```python
from build123d import *

# Parameters (mm, degrees)
BOSS_EXTRUDE1_DEPTH     = 3.7
CHAMFER1_SIZE           = 0.9
CHAMFER1_SIZE2          = 2
CHAMFER2_SIZE           = 2
CHAMFER2_SIZE2          = 0.9
CHAMFER4_SIZE           = 0.9
CHAMFER4_SIZE2          = 2
CHAMFER5_SIZE           = 2
CHAMFER5_SIZE2          = 0.9
CUT_EXTRUDE2_DEPTH      = 1
CUT_EXTRUDE2_DEPTH_BACK = 4.7
CUT_EXTRUDE4_DEPTH      = 1
CUT_EXTRUDE4_DEPTH_BACK = 4.7


with BuildPart() as part:
    # Sketch1 → Boss-Extrude1 (new body)
    with BuildSketch(Plane.XY):
        Polygon((2.936521739, 23.386304348), (2.936521739, -12.613695652), (-3.203478261, -17.151956522), (-3.203478261, 18.848043478), align=None)
    extrude(amount=BOSS_EXTRUDE1_DEPTH)

    # Chamfer1
    chamfer1_edges = [part.edges().sort_by_distance(p)[0] for p in [
        (-0.133478261, 21.117173913, 3.7),
    ]]
    chamfer1_side = [part.faces().sort_by_distance(p)[0] for p in [
        (-0.133478261, 21.117173913, 1.85),
    ]]
    chamfer(chamfer1_edges, length=CHAMFER1_SIZE, length2=CHAMFER1_SIZE2, reference=chamfer1_side[0])

    # Chamfer2
    chamfer2_edges = [part.edges().sort_by_distance(p)[0] for p in [
        (-0.133478261, 21.117173913, 0),
    ]]
    chamfer2_side = [part.faces().sort_by_distance(p)[0] for p in [
        (-0.133478261, 3.117173913, 0),
    ]]
    chamfer(chamfer2_edges, length=CHAMFER2_SIZE, length2=CHAMFER2_SIZE2, reference=chamfer2_side[0])

    # Chamfer4
    chamfer4_edges = [part.edges().sort_by_distance(p)[0] for p in [
        (-0.133478261, -14.882826087, 3.7),
    ]]
    chamfer4_side = [part.faces().sort_by_distance(p)[0] for p in [
        (-0.133478261, -14.882826087, 1.85),
    ]]
    chamfer(chamfer4_edges, length=CHAMFER4_SIZE, length2=CHAMFER4_SIZE2, reference=chamfer4_side[0])

    # Chamfer5
    chamfer5_edges = [part.edges().sort_by_distance(p)[0] for p in [
        (-0.133478261, -14.882826087, 0),
    ]]
    chamfer5_side = [part.faces().sort_by_distance(p)[0] for p in [
        (-0.133478261, 1.873665248, 0),
    ]]
    chamfer(chamfer5_edges, length=CHAMFER5_SIZE, length2=CHAMFER5_SIZE2, reference=chamfer5_side[0])

    # Sketch2 → Cut-Extrude2 (cut, two sides)
    with BuildSketch(Plane.XY.offset(3.7)) as cut_extrude2_sk:
        Polygon((-58.837345155, 2.711026149), (-3.203478261, 2.711026149), (-2.653478261, 2.711026149), (-2.653478261, 1.411026149), (-3.203478261, 1.411026149), (-58.837345155, 1.411026149), (-170.105078945, 1.411026149), (-170.105078945, 2.711026149), align=None)
    extrude(amount=CUT_EXTRUDE2_DEPTH, mode=Mode.SUBTRACT)
    extrude(cut_extrude2_sk.sketch, amount=-CUT_EXTRUDE2_DEPTH_BACK, mode=Mode.SUBTRACT)

    # Sketch3 → Cut-Extrude4 (cut, two sides)
    with BuildSketch(Plane.XY.offset(3.7)) as cut_extrude4_sk:
        Polygon((58.570388634, 2.711026149), (2.936521739, 2.711026149), (2.386521739, 2.711026149), (2.386521739, 1.411026149), (2.936521739, 1.411026149), (58.570388634, 1.411026149), (169.838122423, 1.411026149), (169.838122423, 2.711026149), align=None)
    extrude(amount=CUT_EXTRUDE4_DEPTH, mode=Mode.SUBTRACT)
    extrude(cut_extrude4_sk.sketch, amount=-CUT_EXTRUDE4_DEPTH_BACK, mode=Mode.SUBTRACT)


solid = part.part
```
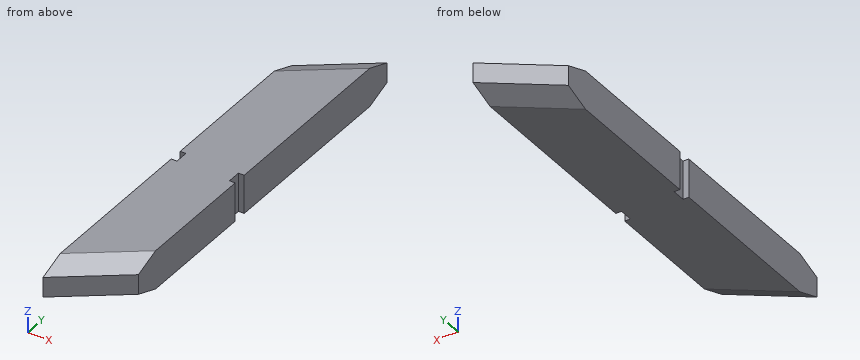
Work out the finished part from the listing and answer in its coordinate system (mm). Coordinates: 2 decimals unless noted, no trailing zeros. Order: outer loops, then holes, each group sorted by start corner. A loop starts at its lowest first (then second) coordinate and runs counter-clockwise, first axis right, second up. Notation, with made-up numbers: (58.25, -5) - (77.25, -5) arc R21 cw to (77.25, 26) - close; hole circle Ø8 at (64, 56). An arc over 180 degrees is marked (long way). Answer as a JSON object with one key per item and string values.
1. Consider line 1 (Y direction, x = 2.25, z = 1.1); line 2 (X direction, y = -13, z = 2.35); line 3 (Z direction, x = -0.5, y = -13). Determine where each line is inside the solid, lowest interval first.
Output values:
{"line 1": "y = -13.12 to 22.88", "line 2": "x = -3.2 to 2.41", "line 3": "z = 0.12 to 3.58"}
2. Find section B-B on x = -0.25. Determine the outline of the cut face in (y, z).
Output values:
{"outline": "(-14.97, 0.9) - (-12.48, 0) - (18.54, 0) - (21.03, 0.9) - (21.03, 2.8) - (18.54, 3.7) - (-12.48, 3.7) - (-14.97, 2.8) - close"}
3. Find section C-C on y = 20. Determine the outline of the cut face in (x, z), plus the area to 3 significant figures.
Output values:
{"outline": "(-1.64, 0.9) - (1.72, 0) - (2.94, 0) - (2.94, 3.7) - (1.72, 3.7) - (-1.64, 2.8) - close", "area": "13.9 mm²"}
4. Each of these flat-tipped pins is pushed along its axis until it touches: P1, Ø1.4, axis at y = 2, z = 2.5, coming from the +X side; P2, Ø0.6, axis at y = 2, z = 2, coming from the -X side. Where does it stop, or does it pass through?
Output values:
{"P1": "stops at x = 2.94", "P2": "stops at x = -2.65"}
5. Find section A-A on z = 1.4. Determine the outline of the cut face in (x, y), plus the area to 3 significant figures.
Output values:
{"outline": "(-3.2, -17.15) - (2.94, -12.61) - (2.94, 1.41) - (2.39, 1.41) - (2.39, 2.71) - (2.94, 2.71) - (2.94, 23.39) - (-3.2, 18.85) - (-3.2, 2.71) - (-2.65, 2.71) - (-2.65, 1.41) - (-3.2, 1.41) - close", "area": "220 mm²"}
6. Find section D-D on z = 3.3. Determine the outline of the cut face in (x, y), plus the area to 3 significant figures.
Output values:
{"outline": "(-3.2, -15.77) - (2.94, -11.23) - (2.94, 1.41) - (2.39, 1.41) - (2.39, 2.71) - (2.94, 2.71) - (2.94, 22) - (-3.2, 17.47) - (-3.2, 2.71) - (-2.65, 2.71) - (-2.65, 1.41) - (-3.2, 1.41) - close", "area": "203 mm²"}
